```python
from build123d import *

# Parameters (mm, degrees)
ESQUISSE1_R        = 80
ESQUISSE1_R_2      = 57
BOSS_EXTRU_1_DEPTH = 46.43


with BuildPart() as part:
    # Esquisse1 → Boss.-Extru.1 (new body)
    with BuildSketch(Plane.XY):
        Circle(ESQUISSE1_R)
        Circle(ESQUISSE1_R_2, mode=Mode.SUBTRACT)
    extrude(amount=BOSS_EXTRU_1_DEPTH)

    # Esquisse2 → Révolution1 (revolve)
    with BuildSketch(Plane(origin=(0, 0, 0), x_dir=(0, 0, -1), z_dir=(1, 0, 0)), mode=Mode.PRIVATE) as r_volution1_sk:
        with BuildLine():
            Line((0, 57), (0.689038023, 57))
            ThreePointArc((0.689038023, 57), (5.003069609, 58.786930391), (6.79, 63.100961977))
            Line((6.79, 63.100961977), (6.79, 64))
            Line((6.79, 64), (6.79, 71.015274994))
            add(Edge.make_bspline(
                [(6.79, 71.015274994), (6.446653278, 77.904299494), (4.024026126, 79.849265176), (0, 80)],
                knots=[0, 0, 0, 0, 1, 1, 1, 1], degree=3))
            Line((0, 80), (0, 57))
        make_face()
        with BuildLine():
            Line((-46.43, 57), (-47.119038023, 57))
            ThreePointArc((-47.119038023, 57), (-51.433069609, 58.786930391), (-53.22, 63.100961977))
            Line((-53.22, 63.100961977), (-53.22, 64))
            Line((-53.22, 64), (-53.22, 71.015274994))
            add(Edge.make_bspline(
                [(-53.22, 71.015274994), (-52.876653278, 77.904299494), (-50.454026126, 79.849265176), (-46.43, 80)],
                knots=[0, 0, 0, 0, 1, 1, 1, 1], degree=3))
            Line((-46.43, 80), (-46.43, 57))
        make_face()
    revolve(r_volution1_sk.sketch.rotate(Axis((0, 0, 0), (0, 0, 1)), 90), axis=Axis((0, 0, 0), (0, 0, 1)))


solid = part.part
```
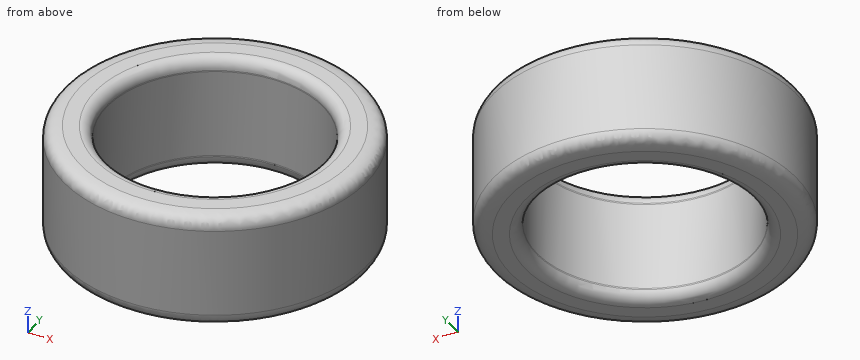
Design review of the part built by this model. Coordinates are the model's own, in mm. Round coordinates to 2 decimals unless told otherwise and drop trailing zeros. Order: outer loops, then holes, each group sorted by start corner. A loop starts at its lowest first (then second) coordinate and runs counter-clockwise, first axis right, second up. Notation, with made-up numbers: (5, 69.5) - (10, 69.5) arc R23 cw to (10, 86.5) - close; hole circle Ø4 at (-33, -38). An arc over 180 degrees is marked (long way). One line per question, with ' | ' between items.
Item 1: For P1, Ø3, axis at y = 5, z = 8, coming from the -X side; P2, Ø3, axis at y = -63.5, z = 15, coming from the +X side; P3, Ø4, axis at x = -15, z = 16.5, coming from the -Y side, all flat-tipped, find the tip position at first contact; note any pin that passes through.
Checks:
P1: x = -79.92 | P2: x = 50.56 | P3: y = -78.94
Item 2: Take a section at A-A, the plane z = 26. Write out the cut boundary in (x, y).
Checks:
outline: circle Ø160 at (0, 0); hole circle Ø114 at (0, 0)
Item 3: Wall thickness on line 1 (Y direction, x = 0, z = 24.5); line 2 (Y direction, x = 7, z = 49); line 3 (X direction, y = -14, z = 42): over which ranges is each line inside the solid? List them lowest first. Write a range as [from, to].
Checks:
line 1: [-80, -57], [57, 80] | line 2: [-79.25, -56.87], [56.87, 79.25] | line 3: [-78.77, -55.25], [55.25, 78.77]
